Could you check a few things on this model? Use its own coordinates, in mm. Face numbers are marked on the shaded views. A direction names the side the tool comes from. Round coordinates to 2 decimals unless told otherwise and drop trailing zeros. Loops run counter-clockwise (first coordinate to the right, second up) from the corner with the lowest first, then second, coordinate; pieces in that order, holes last. Notation, with made-up numbers: (31.25, -5) -> (63.25, -5) arc R9 cw to (63.25, -1) -> close; hole circle Ø1 at (77, -24). An arc over 180 degrees is marked (long way). One line per item, written item: value.
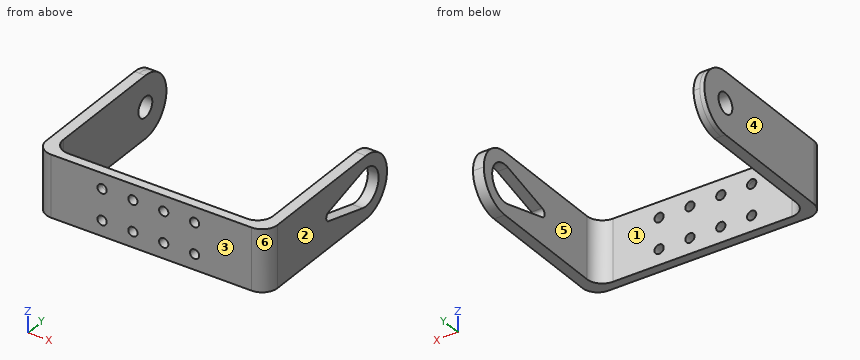
```python
from build123d import *

# Parameters (mm, degrees)
SKETCH_2_R          = 1.5
EXTRUDE_1_DEPTH     = 2
SKETCH_3_W          = 2
SKETCH_3_H          = 20
SKETCH_3_W_2        = 3.5
EXTRUDE_2_DEPTH     = 55
SKETCH_9_R          = 6
CUT_EXTRUDE_1_DEPTH = 87
SKETCH_7_R          = 6
SKETCH_7_R_2        = 3.3
EXTRUDE_3_DEPTH     = 2
SKETCH_10_R         = 3.3
EXTRUDE_4_DEPTH     = 1.5
SKETCH_11_W         = 68
SKETCH_11_H         = 20
SKETCH_11_R         = 1.5
SKETCH_11_R_2       = 1.498871695
EXTRUDE_5_DEPTH     = 1
FILLET_6_R          = 5
FILLET_7_R          = 5
FILLET_8_R          = 5
CUT_EXTRUDE_2_DEPTH = 3.5


with BuildPart() as part:
    # 스케치2 → 보스-돌출1 (new body)
    with BuildSketch(Plane(origin=(0, 0, 0), x_dir=(1, 0, 0), z_dir=(0, 1, 0))):
        Polygon((35, -10), (-35, -10), (-35, 10), (35, 10), (38.5, 10), (38.5, -10), align=None)
        with Locations((-15, 5)):
            Circle(SKETCH_2_R, mode=Mode.SUBTRACT)
        with Locations((-5, 5)):
            Circle(SKETCH_2_R, mode=Mode.SUBTRACT)
        with Locations((-15, -5)):
            Circle(SKETCH_2_R, mode=Mode.SUBTRACT)
        with Locations((-5, -5)):
            Circle(SKETCH_2_R, mode=Mode.SUBTRACT)
        with Locations((15, -5)):
            Circle(SKETCH_2_R, mode=Mode.SUBTRACT)
        with Locations((5, -5)):
            Circle(SKETCH_2_R, mode=Mode.SUBTRACT)
        with Locations((5, 5)):
            Circle(SKETCH_2_R, mode=Mode.SUBTRACT)
        with Locations((15, 5)):
            Circle(SKETCH_2_R, mode=Mode.SUBTRACT)
    extrude(amount=EXTRUDE_1_DEPTH)

    # 스케치3 → 보스-돌출2 (add)
    with BuildSketch(Plane(origin=(0, 2, 0), x_dir=(1, 0, 0), z_dir=(0, 1, 0))):
        with Locations((-34, 0)):
            Rectangle(SKETCH_3_W, SKETCH_3_H)
        with Locations((36.75, 0)):
            Rectangle(SKETCH_3_W_2, SKETCH_3_H)
    extrude(amount=EXTRUDE_2_DEPTH)

    # 스케치9 → 컷-돌출1 (cut)
    with BuildSketch(Plane(origin=(38.5, 0, 0), x_dir=(0, 0, -1), z_dir=(1, 0, 0))):
        with BuildLine():
            Line((10, 57), (0, 57))
            ThreePointArc((0, 57), (7.071067812, 54.071067812), (10, 47))
            Line((10, 47), (10, 57))
        make_face()
        with BuildLine():
            Line((-10, 57), (-10, 47))
            ThreePointArc((-10, 47), (-7.071067812, 54.071067812), (0, 57))
            Line((0, 57), (-10, 57))
        make_face()
        with Locations((0, 47)):
            Circle(SKETCH_9_R)
    extrude(amount=-CUT_EXTRUDE_1_DEPTH, mode=Mode.SUBTRACT)

    # 스케치7 → 보스-돌출3 (add)
    with BuildSketch(Plane.ZY.offset(35)):
        with Locations((0, 47)):
            Circle(SKETCH_7_R)
        with Locations((0, 47)):
            Circle(SKETCH_7_R_2, mode=Mode.SUBTRACT)
    extrude(amount=-EXTRUDE_3_DEPTH)

    # 스케치10 → 보스-돌출4 (add)
    with BuildSketch(Plane.ZY.offset(35)):
        with BuildLine():
            ThreePointArc((-10, 47), (0, 57), (10, 47))
            Line((10, 47), (10, 0))
            Line((10, 0), (-10, 0))
            Line((-10, 0), (-10, 47))
        make_face()
        with Locations((0, 47)):
            Circle(SKETCH_10_R, mode=Mode.SUBTRACT)
    extrude(amount=EXTRUDE_4_DEPTH)

    # 스케치11 → 보스-돌출5 (add)
    with BuildSketch(Plane(origin=(0, 2, 0), x_dir=(1, 0, 0), z_dir=(0, 1, 0))):
        with Locations((1, 0)):
            Rectangle(SKETCH_11_W, SKETCH_11_H)
        with Locations((-15, 5)):
            Circle(SKETCH_11_R, mode=Mode.SUBTRACT)
        with Locations((-5, 5)):
            Circle(SKETCH_11_R, mode=Mode.SUBTRACT)
        with Locations((5, 5)):
            Circle(SKETCH_11_R, mode=Mode.SUBTRACT)
        with Locations((15, 5)):
            Circle(SKETCH_11_R, mode=Mode.SUBTRACT)
        with Locations((15, -5)):
            Circle(SKETCH_11_R, mode=Mode.SUBTRACT)
        with Locations((5, -5)):
            Circle(SKETCH_11_R, mode=Mode.SUBTRACT)
        with Locations((-5, -5)):
            Circle(SKETCH_11_R, mode=Mode.SUBTRACT)
        with Locations((-15, -5)):
            Circle(SKETCH_11_R_2, mode=Mode.SUBTRACT)
    extrude(amount=EXTRUDE_5_DEPTH)

    # 필렛6
    fillet_6_edges = [part.edges().sort_by_distance(p)[0] for p in [
        (-33, 3, 0),
    ]]
    fillet(fillet_6_edges, radius=FILLET_6_R)

    # 필렛7
    fillet_7_edges = [part.edges().sort_by_distance(p)[0] for p in [
        (35, 3, 0),
    ]]
    fillet(fillet_7_edges, radius=FILLET_7_R)

    # 필렛8
    fillet_8_edges = [part.edges().sort_by_distance(p)[0] for p in [
        (-36.5, 0, 0),
        (38.5, 0, 0),
    ]]
    fillet(fillet_8_edges, radius=FILLET_8_R)

    # 스케치12 → 컷-돌출2 (cut)
    with BuildSketch(Plane(origin=(38.5, 0, 0), x_dir=(0, 0, -1), z_dir=(1, 0, 0))):
        with BuildLine():
            ThreePointArc((-1.448888739, 29.225106559), (0, 28.113335127), (1.448888739, 29.225106559))
            Line((1.448888739, 29.225106559), (5.795554958, 45.447085729))
            ThreePointArc((5.795554958, 45.447085729), (0, 41), (-5.795554958, 45.447085729))
            Line((-5.795554958, 45.447085729), (-1.448888739, 29.225106559))
        make_face()
    extrude(amount=-CUT_EXTRUDE_2_DEPTH, mode=Mode.SUBTRACT)


solid = part.part
```
(1) For pin 1 Ø5 at (x, z) = (-5, -5) entering from +Y, with a flat end and sliding along its axis, tell me the tip position at first contact or that it passes through.
Results below:
pin 1: stops at y = 3
(2) Imagine slicing it at C-C on z = -5. Give the number of separate pieces and of enclosed holes in the cut face, then the cut area to 3 significant figures.
Results below:
separate pieces: 6
enclosed holes: 0
area: 530 mm²
(3) On a 3-axis mill with a long thin cutter (end or side, diameter ignored), from which of +Z, -Z, +X, -X, +Y, -Y can I reach the whole of each face in a straight line? I mean the marked faces 1 and 2. Say none if no direction works.
Results below:
face 1: +Z, -Z, +Y
face 2: +Z, -Z, +X, +Y, -Y
(4) We'd pull the mould along X, two halves only. Please class the marked faces 3, 4, 5 and 6: +X half, -X half, draft (parallel to the pull), parting line (faces both ways), or undercut.
Results below:
face 3: draft
face 4: -X half
face 5: undercut
face 6: +X half
(5) Imagine slicing it at B-B on y = 12.5. Write out the boundary of the cut face in (x, z).
Results below:
outline: (-36.5, -10) -> (-33, -10) -> (-33, 10) -> (-36.5, 10) -> close; (35, -10) -> (38.5, -10) -> (38.5, 10) -> (35, 10) -> close
(6) Imagine slicing it at A-A on x = -5. Write out the boundary of the cut face in (y, z).
Results below:
outline: (0, -10) -> (3, -10) -> (3, -6.5) -> (0, -6.5) -> close; (0, -3.5) -> (3, -3.5) -> (3, 3.5) -> (0, 3.5) -> close; (0, 6.5) -> (3, 6.5) -> (3, 10) -> (0, 10) -> close
(7) Please list where these lines run through material, in increasing order: L1, parallel to Z at x = 15, y = 1.55; L2, parallel to X at y = 15, z = 9.25; L3, parallel to Z at x = 35.85, y = 47.
Results below:
L1: z = -10 to -6.5, -3.5 to 3.5, 6.5 to 10
L2: x = -36.5 to -33, 35 to 38.5
L3: z = -10 to -6, 6 to 10
